```python
from build123d import *

# Parameters (mm, degrees)
SKIZZE1_W                       = 6
SKIZZE1_H                       = 6
SKIZZE1_W_2                     = 5
SKIZZE1_H_2                     = 5
AUFSATZ_LINEAR_AUSTRAGEN1_DEPTH = 3
VERRUNDUNG1_R                   = 1
SKIZZE2_W                       = 1.5
SKIZZE2_H                       = 2
SKIZZE2_W_2                     = 2
SKIZZE2_H_2                     = 1.5
AUFSATZ_LINEAR_AUSTRAGEN2_DEPTH = 1
VERRUNDUNG2_R                   = 1.5
VERRUNDUNG3_R                   = 0.5
M1_6_GEWINDEBOHRUNG5_D          = 1.25
M1_6_GEWINDEBOHRUNG5_DEPTH      = 3.09
M1_6_GEWINDEBOHRUNG5_TIP        = 0.625


with BuildPart() as part:
    # Skizze1 → Aufsatz-Linear austragen1 (new body)
    with BuildSketch(Plane.XY):
        Rectangle(SKIZZE1_W, SKIZZE1_H)
        Rectangle(SKIZZE1_W_2, SKIZZE1_H_2, mode=Mode.SUBTRACT)
        Polygon((1.939339828, 4.060660172), (0.878679656, 3), (3, 3), align=None)
        Polygon((4.060660172, 1.939339828), (3, 3), (3, 0.878679656), align=None)
    extrude(amount=AUFSATZ_LINEAR_AUSTRAGEN1_DEPTH)

    # Verrundung1
    verrundung1_edges = [part.edges().sort_by_distance(p)[0] for p in [
        (-2.5, 2.5, 1.5),
        (-2.5, -2.5, 1.5),
        (2.5, -2.5, 1.5),
        (2.5, 2.5, 1.5),
    ]]
    fillet(verrundung1_edges, radius=VERRUNDUNG1_R)

    # Skizze2 → Aufsatz-Linear austragen2 (add)
    with BuildSketch(Plane.XY):
        with Locations((-0.75, 4)):
            Rectangle(SKIZZE2_W, SKIZZE2_H)
        with Locations((0, -4)):
            Rectangle(SKIZZE2_W, SKIZZE2_H)
        with Locations((-4, 0)):
            Rectangle(SKIZZE2_W_2, SKIZZE2_H_2)
        with Locations((4, -0.75)):
            Rectangle(SKIZZE2_W_2, SKIZZE2_H_2)
    extrude(amount=AUFSATZ_LINEAR_AUSTRAGEN2_DEPTH)

    # Verrundung2
    verrundung2_edges = [part.edges().sort_by_distance(p)[0] for p in [
        (3, -3, 1.5),
        (-3, -3, 1.5),
        (-3, 3, 1.5),
    ]]
    fillet(verrundung2_edges, radius=VERRUNDUNG2_R)

    # Verrundung3
    verrundung3_edges = [part.edges().sort_by_distance(p)[0] for p in [
        (3, 0, 0.5),
        (3, -1.5, 0.5),
        (0.878679656, 3, 1.5),
        (3, 0.878679656, 1.5),
        (-1.5, 3, 0.5),
        (0, 3, 0.5),
        (0.75, -3, 0.5),
        (-0.75, -3, 0.5),
        (-3, -0.75, 0.5),
        (-3, 0.75, 0.5),
    ]]
    fillet(verrundung3_edges, radius=VERRUNDUNG3_R)

    # M1.6 Gewindebohrung5
    with Locations(Plane(origin=(3, 3, 0), x_dir=(0.707106781, -0.707106781, 0), z_dir=(0.707106781, 0.707106781, 0))):
        with Locations((0, -1.5)):
            Hole(M1_6_GEWINDEBOHRUNG5_D / 2, depth=M1_6_GEWINDEBOHRUNG5_DEPTH)
            with Locations((0, 0, -(M1_6_GEWINDEBOHRUNG5_DEPTH + M1_6_GEWINDEBOHRUNG5_TIP / 2))):  # 90° drill point
                Cone(0, M1_6_GEWINDEBOHRUNG5_D / 2, M1_6_GEWINDEBOHRUNG5_TIP, mode=Mode.SUBTRACT)


solid = part.part
```
Check sheet for the modelled part. Datum: model origin and axes. Units: mm. A direction names the side the tool comes from. Round coordinates to 2 decimals unless told otherwise and drop trailing zeros. Order: outer loops, then holes, each group sorted by start corner. A loop starts at its lowest first (then second) coordinate and runs counter-clockwise, first axis right, second up.
1) Go/stop test with flat-tipped pins: pin 1 Ø1.5 at (y, z) = (-3, 1.5) entering from -X; pin 2 Ø1.5 at (x, y) = (0.5, 0.5) entering from +Z; pin 3 Ø1 at (x, z) = (-3, 2.5) entering from +Y; pin 4 Ø1 at (x, y) = (-4, 0) entering from +Z. Record where each tip stops, or that it passes through.
2) Scan lines: line 1 (Y direction, x = -0.25, z = 2.35); line 2 (X direction, y = 3.75, z = 0.2). Record each from-to range of solid material in increasing order.
3) Section check C-C (y = -2). Record the boundary of the cut face in (x, z).
4) Section check A-A (z = 2.65). Record the boundary of the cut face in (x, y).
5) Tool access check on faces 1 (the flat face through (-5, 0, 0.5)), 2 (the flat face through (4.2, -1.5, 0.5)), 3 (the flat face through (-1, 4, 1)), 4 (the flat face through (-2.5, 0, 1)), 5 (the flat face through (-0.75, -4.3, 0.5)). Record the directions out of +Z, -Z, +X, -X, +Y, -Y that give a thin tool (end or side, any length) a straight path to the whole face; none if there is none.
6) Mould release check, pull along Y, two halves, no side actions. Record for faces 6 (the flat face through (3, 0, 0)), 7 (the flat face through (0, 2.5, 1)), 8 (the flat face through (1.49, 3.61, 1.48)): +Y half, -Y half, draft (parallel to the pull), parting line (faces both ways), or undercut.
7) Section check B-B (x = -0.25). Record the boundary of the cut face in (y, z).
Result:
1. pin 1: stops at x = -2.8
1. pin 2: passes through
1. pin 3: stops at y = 2.62
1. pin 4: stops at z = 1
2. line 1: y = -3 to -2.5, 2.5 to 3
2. line 2: x = -1.5 to 0, 1.63 to 2.25
3. outline: (-2.91, 0) - (-2.37, 0) - (-2.37, 3) - (-2.91, 3) - close; (2.37, 0) - (2.91, 0) - (2.91, 3) - (2.37, 3) - close
4. outline: (-3, -1.5) arc R1.5 ccw to (-1.5, -3) - (1.5, -3) arc R1.5 ccw to (3, -1.5) - (3, 0.67) arc R0.5 cw to (3.15, 1.03) - (4.06, 1.94) - (1.94, 4.06) - (1.03, 3.15) arc R0.5 cw to (0.67, 3) - (-1.5, 3) arc R1.5 ccw to (-3, 1.5) - close; hole (-2.5, -1.5) arc R1 ccw to (-1.5, -2.5) - (1.5, -2.5) arc R1 ccw to (2.5, -1.5) - (2.5, 1.5) arc R1 ccw to (1.5, 2.5) - (-1.5, 2.5) arc R1 ccw to (-2.5, 1.5) - close
5. face 1: +Z, -Z, -X, +Y, -Y
5. face 2: +Z, -Z, +X, -Y
5. face 3: +Z, -X, +Y
5. face 4: +Z, -Z
5. face 5: +Z, -Z, -X, -Y
6. face 6: draft
6. face 7: undercut
6. face 8: +Y half
7. outline: (-5, 0) - (-2.5, 0) - (-2.5, 3) - (-3, 3) - (-3, 1) - (-5, 1) - close; (2.5, 0) - (5, 0) - (5, 1) - (3, 1) - (3, 3) - (2.5, 3) - close
